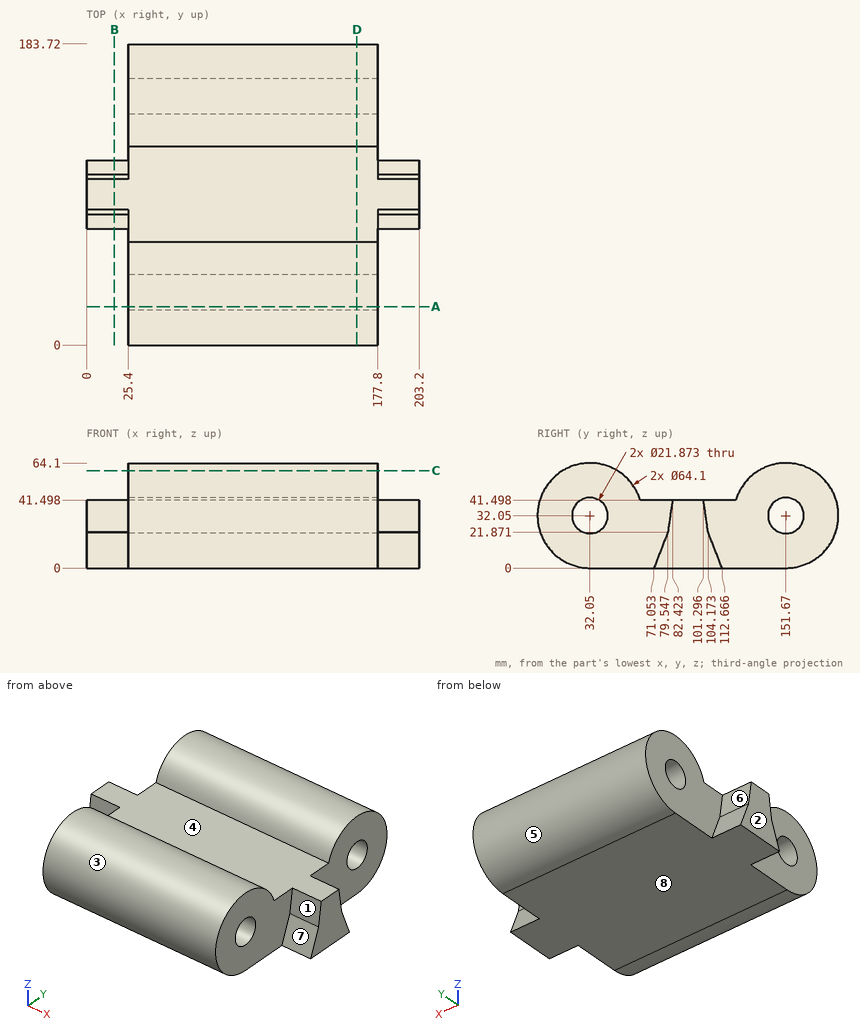
Drawing for the job (mm, zero at the part's lowest x, y, z). A direction names the side the tool comes from. Coordinates: 2 decimals unless noted, no trailing zeros. Order: outer loops, then holes, each group sorted by start corner. A loop starts at its lowest first (then second) coordinate and runs counter-clockwise, first axis right, second up. Notation, with made-up numbers: (63.25, 53.25) -> (79.25, 53.25) arc R8 ccw to (79.25, 62.25) -> close; hole circle Ø6 at (-11.75, 88.5). An arc over 180 degrees is marked (long way). One line per item, written item: value.
(1) Slice it at A-A, the plane y = 23.5. List the corners of the cut face in (x, z), plus the area to 3 significant figures.
Checked values:
outline: (25.4, 1.16) -> (177.8, 1.16) -> (177.8, 25.23) -> (25.4, 25.23) -> close; (25.4, 38.87) -> (177.8, 38.87) -> (177.8, 62.94) -> (25.4, 62.94) -> close
area: 7,340 mm2
(2) Slice it at D-D, the plane x = 165. Count the separate pieces of the cut face and the enclosed holes in it, plus the area to 3 significant figures.
Checked values:
separate pieces: 1
enclosed holes: 2
area: 8,460 mm2
(3) Drop flat-ended pins along their axis: pin 1 Ø3 at (x, z) = (148, 7.5) entering from -Y; pin 2 Ø17.5 at (y, z) = (151.67, 32.05) entering from +X; pin 3 Ø1 at (x, y) = (129, 135) entering from +Z; pin 4 Ø1 at (y, z) = (29, 15) entering from -X. Give the stop position or say it passes through.
Checked values:
pin 1: y = 9.78
pin 2: through
pin 3: z = 59.72
pin 4: x = 25.4
(4) Tool access for the marked faces 4, 5, 6, 7 and 8: list every direction of +Z, -Z, +X, -X, +Y, -Y with a clear straight run to the whole face (end or side of a thin tool).
Checked values:
face 4: +Z, +X, -X
face 5: +X, -X
face 6: +Z, -X, +Y
face 7: +Z, +X, -Y
face 8: -Z, +X, -X, +Y, -Y
(5) Slice it at C-C, the plane z = 59.5. List the corners of the cut face in (x, y), plus the area to 3 significant figures.
Checked values:
outline: (25.4, 15.51) -> (177.8, 15.51) -> (177.8, 48.59) -> (25.4, 48.59) -> close; (25.4, 135.13) -> (177.8, 135.13) -> (177.8, 168.21) -> (25.4, 168.21) -> close
area: 10,100 mm2
(6) Mould opens along Y. For the marked faces 1, 2 and 3 say: pulls with the +Y half, pulls with the -Y half, needs draft (parallel to the pull), parting line crosses it, or undercut.
Checked values:
face 1: pulls with the -Y half
face 2: needs draft
face 3: undercut
(7) Slice it at B-B, the plane x = 17. List the corners of the cut face in (y, z).
Checked values:
outline: (71.05, 0) -> (112.67, 0) -> (104.17, 21.87) -> (101.3, 41.5) -> (82.42, 41.5) -> (79.55, 21.87) -> close
(8) Probe line 1 (Y direction, x = 92.5, z = 39) (1 decimal); line 2 (Y direction, x = 151.5, z = 24.5) (1 decimal); line 3 (X direction, y = 14.5, z = 13.5). List the from-to ranges inside material, lowest first. Write a range as [from, to].
Checked values:
line 1: [0.8, 23.6], [40.5, 143.2], [160.1, 183]
line 2: [0.9, 24.1], [40, 143.8], [159.6, 182.8]
line 3: [25.4, 177.8]
